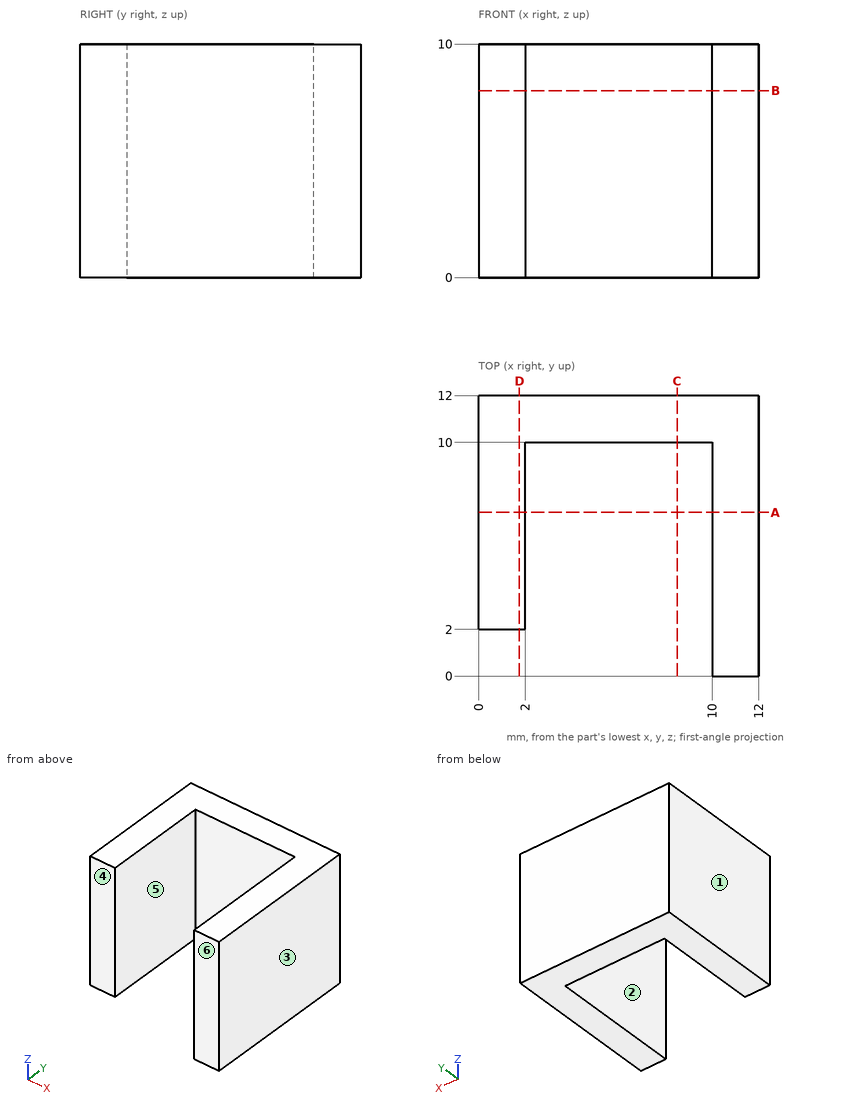
Could you check a few things on this drawing? It's one solid part, dimensions in mm from its lowest x, y, z. A direction names the side the tool comes from. Round coordinates to 2 decimals unless told otherwise and drop trailing zeros. Write each loop counter-clockwise with the first axis right and the second up, starting at its lowest first coordinate (ties: lowest second). Pieces come first, ordered by that corner, then holes. Notation, with made-up numbers: (68, 89) -> (114, 89) arc R16 cw to (114, 112) -> close; hole circle Ø4 at (-14.5, 27.25). An arc over 180 degrees is marked (long way). Use a Markdown table: item, result.
1. If we section it at D-D (x = 1.75): List the corners of the cut face in (y, z) for me, then the cut area to 3 significant figures.
Answer key:
| item | result |
|---|---|
| outline | (2, 0) -> (12, 0) -> (12, 10) -> (2, 10) -> close |
| area | 100 mm^2 |
2. Which directions (+Z, -Z, +X, -X, +Y, -Y) give clear straight access to the entire face, cutting with the end or side of a thin tool? Please do the marked faces 4, 5 and 6.
Answer key:
| item | result |
|---|---|
| face 4 | +Z, -Z, -X, -Y |
| face 5 | +Z, -Z, -Y |
| face 6 | +Z, -Z, +X, -X, -Y |
3. Please list where these lines run through material, in increasing order: probe 1 along X at (y, z) = (3.25, 6.75); probe 2 along Y at (x, z) = (3.75, 4); probe 3 along Y at (x, z) = (1, 3.75).
Answer key:
| item | result |
|---|---|
| probe 1 | x = 0 to 2, 10 to 12 |
| probe 2 | y = 10 to 12 |
| probe 3 | y = 2 to 12 |
4. For pin 1 Ø2 at (x, z) = (5, 5) entering from -Y; pin 2 Ø2 at (x, y) = (4, 5) entering from +Z; pin 3 Ø1.6 at (x, z) = (1.5, 4) entering from -Y, each with a flat end and sliding along its axis, tell me the tip position at first contact or that it passes through.
Answer key:
| item | result |
|---|---|
| pin 1 | stops at y = 10 |
| pin 2 | passes through |
| pin 3 | stops at y = 2 |
5. If we section it at B-B (z = 8): List the corners of the cut face in (x, y) for me, then the cut area to 3 significant figures.
Answer key:
| item | result |
|---|---|
| outline | (0, 2) -> (2, 2) -> (2, 10) -> (10, 10) -> (10, 0) -> (12, 0) -> (12, 12) -> (0, 12) -> close |
| area | 60.0 mm^2 |
6. If we section it at A-A (y = 7): List the corners of the cut face in (x, z) for me, then the cut area to 3 significant figures.
Answer key:
| item | result |
|---|---|
| outline | (0, 0) -> (2, 0) -> (2, 10) -> (0, 10) -> close; (10, 0) -> (12, 0) -> (12, 10) -> (10, 10) -> close |
| area | 40.0 mm^2 |
7. We'd pull the mould along X, two halves only. Please class the marked faces 1, 2 and 3: +X half, -X half, draft (parallel to the pull), parting line (faces both ways), or undercut.
Answer key:
| item | result |
|---|---|
| face 1 | -X half |
| face 2 | undercut |
| face 3 | +X half |
8. If we section it at C-C (x = 8.5): List the corners of the cut face in (y, z) for me.
Answer key:
| item | result |
|---|---|
| outline | (10, 0) -> (12, 0) -> (12, 10) -> (10, 10) -> close |
